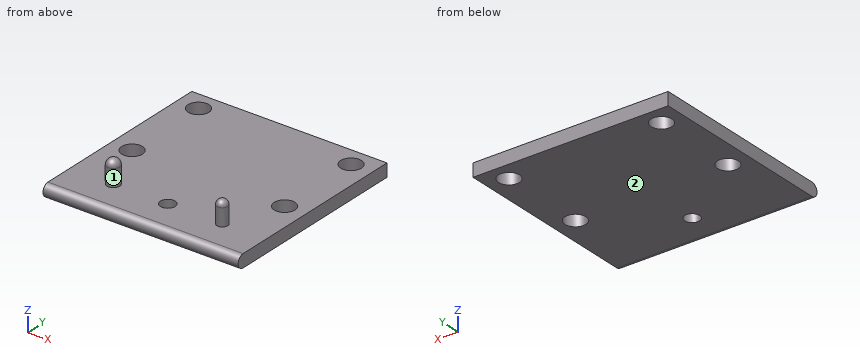
```python
from build123d import *

# Parameters (mm, degrees)
SKETCH1_W            = 44.8
SKETCH1_H            = 2.99
BOSS_EXTRUDE1_DEPTH  = 44.8
FILLET1_RADIUS       = 1.495
FILLET1_LENGTH       = 44.8
M4_CLEARANCE_HOLE1_D = 4.8
M3_CLEARANCE_HOLE1_D = 3.4
SKETCH8_R            = 1.481852537
SKETCH8_R_2          = 1.249642824
BOSS_EXTRUDE2_DEPTH  = 4
REVOLVE1_ANGLE       = 180
REVOLVE2_ANGLE       = 180


with BuildPart() as part:
    # Sketch1 → Boss-Extrude1 (new body)
    with BuildSketch(Plane(origin=(0, 0, 0), x_dir=(1, 0, 0), z_dir=(0, 1, 0))):
        Rectangle(SKETCH1_W, SKETCH1_H)
    extrude(amount=BOSS_EXTRUDE1_DEPTH)

    # Fillet1: full round fillet: the end face becomes a half cylinder, R = half its width
    fillet1_face = Plane((0, 0, 0), x_dir=(-1, 0, 0), z_dir=(0, -1, 0))  # on the end face: x along it, z out of the body
    fillet1_slab = fillet1_face.offset(-FILLET1_RADIUS / 2) * Box(FILLET1_LENGTH, 2 * FILLET1_RADIUS, FILLET1_RADIUS, mode=Mode.PRIVATE)  # the body's end, R deep
    fillet1_round = Plane((0, 1.495, 0), x_dir=(0, -1, 0), z_dir=(-1, 0, 0)) * Cylinder(FILLET1_RADIUS, FILLET1_LENGTH, mode=Mode.PRIVATE)  # its axis R under the face
    add(fillet1_slab - fillet1_round, mode=Mode.SUBTRACT)

    # M4 Clearance Hole1 (through all)
    with Locations(Plane.XY.offset(1.495)):
        with Locations((-17.5, 40.4), (-17.5, 20.4), (17.5, 20.4), (17.5, 40.4)):
            Hole(M4_CLEARANCE_HOLE1_D / 2)

    # M3 Clearance Hole1 (through all)
    with Locations(Plane.XY.offset(1.495)):
        with Locations((0, 8.2)):
            Hole(M3_CLEARANCE_HOLE1_D / 2)

    # Sketch8 → Boss-Extrude2 (add)
    with BuildSketch(Plane.XY.offset(1.495)):
        with Locations(Location((-12.5, 8.2, 0), (0, 0, 180))):
            Circle(SKETCH8_R)
        with Locations(Location((12.5, 8.2, 0), (0, 0, 180))):
            Circle(SKETCH8_R_2)
    extrude(amount=BOSS_EXTRUDE2_DEPTH)

    # Sketch9 → Revolve1 (revolve)
    with BuildSketch(Plane.XY.offset(5.495)):
        with BuildLine():
            Line((-12.5, 9.681852537), (-12.5, 6.718147463))
            ThreePointArc((-12.5, 6.718147463), (-11.018147463, 8.2), (-12.5, 9.681852537))
        make_face()
    revolve(axis=Axis((-12.5, 9.681852537, 5.495), (0, -1, 0)), revolution_arc=REVOLVE1_ANGLE)

    # Sketch10 → Revolve2 (revolve)
    with BuildSketch(Plane.XY.offset(5.495)):
        with BuildLine():
            Line((12.5, 9.449642824), (12.5, 6.950357176))
            ThreePointArc((12.5, 6.950357176), (13.749642824, 8.2), (12.5, 9.449642824))
        make_face()
    revolve(axis=Axis((12.5, 9.449642824, 5.495), (0, -1, 0)), revolution_arc=REVOLVE2_ANGLE)


solid = part.part
```
Verification items for the finished model (mm, model axes). Face numbers are marked on the shaded views. Give positions to 0.01 mm unless a question says otherwise; leave off trailing zeros. Write each loop counter-clockwise with the first axis right and the second up, starting at its lowest first coordinate (ties: lowest second). Pieces come first, ordered by that corner, then holes. Notation, with made-up numbers: (8.5, -10) - (65.5, -10) arc R28 cw to (65.5, 23) - close; hole circle Ø7 at (45.5, -23.5). An arc over 180 degrees is marked (long way). Put each result on its own line as item: value.
Q1. Section check D-D on z = 0. Record the cut outline in (x, y).
Result:
outline: (-22.4, 0) - (22.4, 0) - (22.4, 44.8) - (-22.4, 44.8) - close; hole circle Ø4.8 at (-17.5, 20.4); hole circle Ø4.8 at (-17.5, 40.4); hole circle Ø3.4 at (0, 8.2); hole circle Ø4.8 at (17.5, 20.4); hole circle Ø4.8 at (17.5, 40.4)
Q2. Scan lines: probe 1 along X at (y, z) = (22, 0.25); probe 2 along Y at (x, z) = (-17.5, 0.15); probe 3 along Y at (x, z) = (-16, 1). Record each from-to range of solid material in increasing order. Write a range as from..to.
Result:
probe 1: -22.4..-19.29, -15.71..15.71, 19.29..22.4
probe 2: 0.01..18, 22.8..38, 42.8..44.8
probe 3: 0.38..18.53, 22.27..38.53, 42.27..44.8
Q3. Section check A-A on x = 0. Record the cut outline in (y, z) (3 decimals), and give its area (3 significant figures).
Result:
outline: (1.495, -1.495) - (6.5, -1.495) - (6.5, 1.495) - (1.495, 1.495) arc R1.495 ccw to start; (9.9, -1.495) - (44.8, -1.495) - (44.8, 1.495) - (9.9, 1.495) - close
area: 123 mm2
Q4. Depth check by flat-ended pin: P1, Ø5.5, axis at x = 17.5, y = 20.4, coming from the +Z side (3 decimals); P2, Ø1, axis at x = -5, z = 3.5, coming from the +Y side. Enter the tip coordinate at first touch or a pass-through.
Result:
P1: z = 1.495
P2: through
Q5. Section check C-C on x = -17.5. Record the cut outline in (y, z) (3 decimals), and give its area (3 significant figures).
Result:
outline: (1.495, -1.495) - (18, -1.495) - (18, 1.495) - (1.495, 1.495) arc R1.495 ccw to start; (22.8, -1.495) - (38, -1.495) - (38, 1.495) - (22.8, 1.495) - close; (42.8, -1.495) - (44.8, -1.495) - (44.8, 1.495) - (42.8, 1.495) - close
area: 104 mm2
Q6. Section check B-B on y = 8.2. Record the cut outline in (x, z) (3 decimals), and give its area (3 significant figures).
Result:
outline: (-22.4, -1.495) - (-1.7, -1.495) - (-1.7, 1.495) - (-11.018, 1.495) - (-11.018, 5.495) arc R1.482 ccw to (-13.982, 5.495) - (-13.982, 1.495) - (-22.4, 1.495) - close; (1.7, -1.495) - (22.4, -1.495) - (22.4, 1.495) - (13.75, 1.495) - (13.75, 5.495) arc R1.25 ccw to (11.25, 5.495) - (11.25, 1.495) - (1.7, 1.495) - close
area: 152 mm2
Q7. Mould release check, pull along X, two halves, no side actions. Record for the marked faces 1 and 2: released by +X, released by -X, zero draft, split by the parting line, or undercut.
Result:
face 1: undercut
face 2: zero draft
